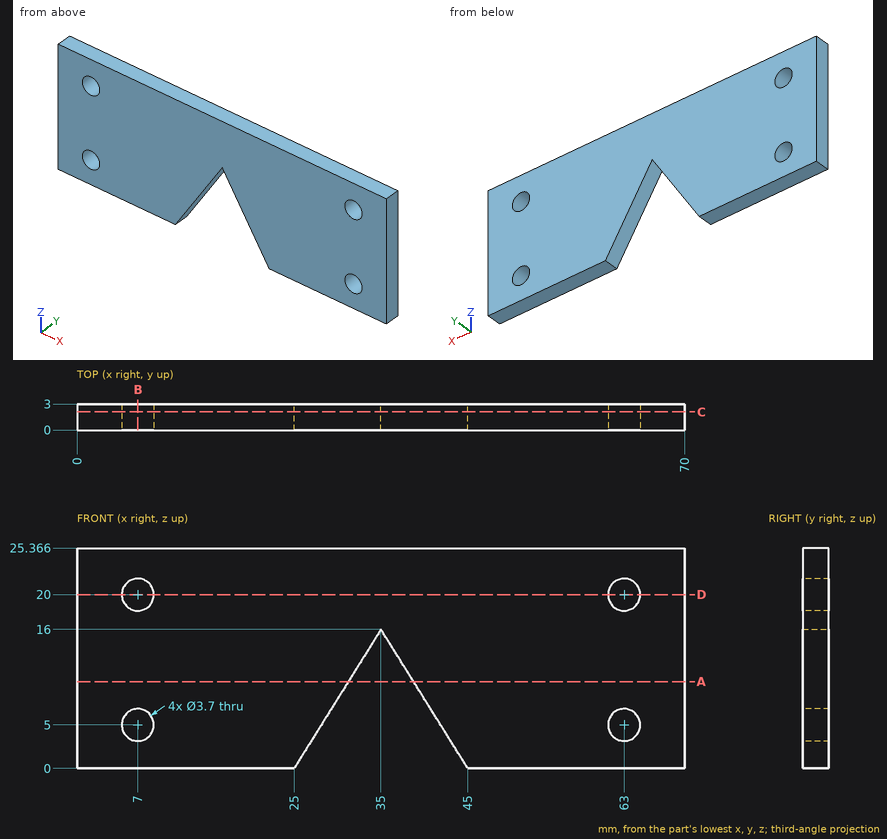
Drawing for the job (mm, zero at the part's lowest x, y, z). Round coordinates to 2 decimals unless told otherwise and drop trailing zeros. Write each loop counter-clockwise with the first axis right and the second up, starting at its lowest first coordinate (ties: lowest second). Pieces come first, ordered by that corner, then holes. Notation, with made-up numbers: M -18,46.25 L 9,46.25 A26 cw 9,83.25 Z; hole C 32.5,47.25 d6. An arc over 180 degrees is marked long. Answer in a Markdown table with one row per item.
1. Flat gauge pin, fed straight in: P1, Ø3.5, axis at x = 7, z = 5, coming from the -Y side. Where does the tip first touch, or does it go through?
Geometry check:
| item | result |
|---|---|
| P1 | through |
2. Saw through at D-D (z = 20). List the corners of the cut face in (x, y), and give its area (3 significant figures).
Geometry check:
| item | result |
|---|---|
| outline | M 0,0 L 5.15,0 L 5.15,3 L 0,3 Z; M 8.85,0 L 61.15,0 L 61.15,3 L 8.85,3 Z; M 64.85,0 L 70,0 L 70,3 L 64.85,3 Z |
| area | 188 mm2 |
3. Saw through at B-B (x = 7). List the corners of the cut face in (y, z).
Geometry check:
| item | result |
|---|---|
| outline | M 0,0 L 3,0 L 3,3.15 L 0,3.15 Z; M 0,6.85 L 3,6.85 L 3,18.15 L 0,18.15 Z; M 0,21.85 L 3,21.85 L 3,25.37 L 0,25.37 Z |
4. Saw through at C-C (y = 2.1). List the corners of the cut face in (x, z), and give its area (3 significant figures).
Geometry check:
| item | result |
|---|---|
| outline | M 0,0 L 25,0 L 35,16 L 45,0 L 70,0 L 70,25.37 L 0,25.37 Z; hole C 7,5 d3.7; hole C 7,20 d3.7; hole C 63,5 d3.7; hole C 63,20 d3.7 |
| area | 1,570 mm2 |
5. Saw through at A-A (z = 10). List the corners of the cut face in (x, y).
Geometry check:
| item | result |
|---|---|
| outline | M 0,0 L 31.25,0 L 31.25,3 L 0,3 Z; M 38.75,0 L 70,0 L 70,3 L 38.75,3 Z |
6. Probe L1, parallel to Z at x = 7, y = 2; L2, parallel to X at y = 2.45, z = 20; L3, parallel to X at y = 2.5, z = 6.25 (1 decimal). List the from-to ranges inside material, lowest first. Write a range as [from, to].
Geometry check:
| item | result |
|---|---|
| L1 | [0, 3.15], [6.85, 18.15], [21.85, 25.37] |
| L2 | [0, 5.15], [8.85, 61.15], [64.85, 70] |
| L3 | [0, 5.6], [8.4, 28.9], [41.1, 61.6], [64.4, 70] |
